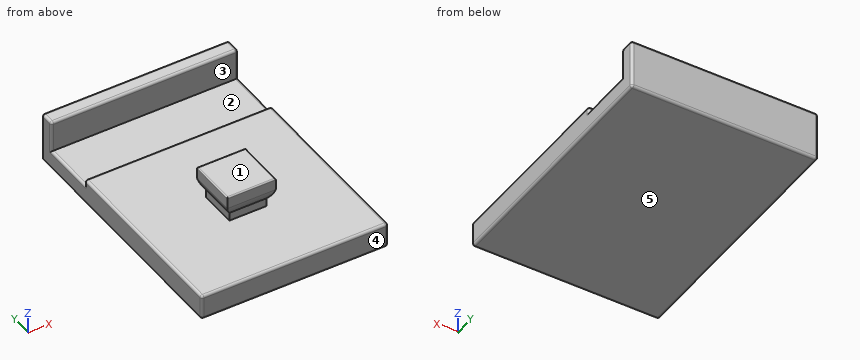
```python
from build123d import *

# Parameters (mm, degrees)
SKETCH_1_W                      = 15
SKETCH_1_H                      = 15
EXTRUDE_1_DEPTH                 = 2
SKETCH_2_W                      = 3
SKETCH_2_H                      = 3
EXTRUDE_2_DEPTH                 = 1
EXTRUDE_3_DEPTH                 = 2
EXTRUDE_3_DEPTH_BACK            = 2
CUT_EXTRUDE_1_REACH             = 12.897
CUT_EXTRUDE_1_DIRECTION_2_REACH = 12.897
FILLET_1_R                      = 0.1
SKETCH_5_W                      = 15
SKETCH_5_H                      = 1.5
EXTRUDE_4_DEPTH                 = 5.5
SKETCH_6_W                      = 15
SKETCH_6_H                      = 1.2
EXTRUDE_5_DEPTH                 = 2.5
FILLET_2_R                      = 0.2


with BuildPart() as part:
    # 草图1 → 凸台-拉伸1 (new body)
    with BuildSketch(Plane.XY):
        Rectangle(SKETCH_1_W, SKETCH_1_H)
    extrude(amount=-EXTRUDE_1_DEPTH)

    # 草图2 → 凸台-拉伸2 (add)
    with BuildSketch(Plane.XY):
        Rectangle(SKETCH_2_W, SKETCH_2_H)
    extrude(amount=EXTRUDE_2_DEPTH)

    # 草图3 → 凸台-拉伸3 (add, two sides: drawn at the far end of the back side and taken through both)
    with BuildSketch(Plane(origin=(0, 0, 0), x_dir=(1, 0, 0), z_dir=(0, 1, 0)).offset(-EXTRUDE_3_DEPTH_BACK)):
        with BuildLine():
            Line((-1.95, -2.5), (1.95, -2.5))
            Line((1.95, -2.5), (1.95, -1.555590279))
            ThreePointArc((1.95, -1.555590279), (1.780042303, -1.088161527), (1.5, -0.677124344))
            Line((1.5, -0.677124344), (-1.5, -0.677124344))
            ThreePointArc((-1.5, -0.677124344), (-1.780042303, -1.088161527), (-1.95, -1.555590279))
            Line((-1.95, -1.555590279), (-1.95, -2.5))
        make_face()
    extrude(amount=EXTRUDE_3_DEPTH + EXTRUDE_3_DEPTH_BACK)

    # 草图4 → 切除-拉伸1 (cut, up to next)
    with BuildSketch(Plane(origin=(0, 0, 0), x_dir=(0, 0, -1), z_dir=(1, 0, 0)), mode=Mode.PRIVATE) as cut_extrude_1_sk1:
        with BuildLine():
            Line((-2.5, 1.95), (-1.555590279, 1.95))
            ThreePointArc((-1.555590279, 1.95), (-1.088161527, 1.780042303), (-0.677124344, 1.5))
            Line((-0.677124344, 1.5), (-0.677124344, 2))
            Line((-0.677124344, 2), (-2.5, 2))
            Line((-2.5, 2), (-2.5, 1.95))
        make_face()
    cut_extrude_1_tool1 = extrude(cut_extrude_1_sk1.sketch, amount=-CUT_EXTRUDE_1_REACH, mode=Mode.PRIVATE) & part.part
    # 草图4 → 切除-拉伸1 (cut, up to next)
    with BuildSketch(Plane(origin=(0, 0, 0), x_dir=(0, 0, -1), z_dir=(1, 0, 0)), mode=Mode.PRIVATE) as cut_extrude_1_sk2:
        with BuildLine():
            Line((-2.5, -2), (-0.677124344, -2))
            Line((-0.677124344, -2), (-0.677124344, -1.5))
            ThreePointArc((-0.677124344, -1.5), (-1.088161527, -1.780042303), (-1.555590279, -1.95))
            Line((-1.555590279, -1.95), (-2.5, -1.95))
            Line((-2.5, -1.95), (-2.5, -2))
        make_face()
    cut_extrude_1_tool2 = extrude(cut_extrude_1_sk2.sketch, amount=-CUT_EXTRUDE_1_REACH, mode=Mode.PRIVATE) & part.part
    add(cut_extrude_1_tool1.solids().sort_by_distance((0, 1.873038, 1.175075))[0], mode=Mode.SUBTRACT)
    add(cut_extrude_1_tool2.solids().sort_by_distance((0, -1.873038, 1.175075))[0], mode=Mode.SUBTRACT)

    # 草图4 → 切除-拉伸1 direction 2 (cut, up to next)
    with BuildSketch(Plane(origin=(0, 0, 0), x_dir=(0, 0, -1), z_dir=(1, 0, 0)), mode=Mode.PRIVATE) as cut_extrude_1_direction_2_sk1:
        with BuildLine():
            Line((-2.5, 1.95), (-1.555590279, 1.95))
            ThreePointArc((-1.555590279, 1.95), (-1.088161527, 1.780042303), (-0.677124344, 1.5))
            Line((-0.677124344, 1.5), (-0.677124344, 2))
            Line((-0.677124344, 2), (-2.5, 2))
            Line((-2.5, 2), (-2.5, 1.95))
        make_face()
    cut_extrude_1_direction_2_tool1 = extrude(cut_extrude_1_direction_2_sk1.sketch, amount=CUT_EXTRUDE_1_DIRECTION_2_REACH, mode=Mode.PRIVATE) & part.part
    # 草图4 → 切除-拉伸1 direction 2 (cut, up to next)
    with BuildSketch(Plane(origin=(0, 0, 0), x_dir=(0, 0, -1), z_dir=(1, 0, 0)), mode=Mode.PRIVATE) as cut_extrude_1_direction_2_sk2:
        with BuildLine():
            Line((-2.5, -2), (-0.677124344, -2))
            Line((-0.677124344, -2), (-0.677124344, -1.5))
            ThreePointArc((-0.677124344, -1.5), (-1.088161527, -1.780042303), (-1.555590279, -1.95))
            Line((-1.555590279, -1.95), (-2.5, -1.95))
            Line((-2.5, -1.95), (-2.5, -2))
        make_face()
    cut_extrude_1_direction_2_tool2 = extrude(cut_extrude_1_direction_2_sk2.sketch, amount=CUT_EXTRUDE_1_DIRECTION_2_REACH, mode=Mode.PRIVATE) & part.part
    add(cut_extrude_1_direction_2_tool1.solids().sort_by_distance((0, 1.873038, 1.175075))[0], mode=Mode.SUBTRACT)
    add(cut_extrude_1_direction_2_tool2.solids().sort_by_distance((0, -1.873038, 1.175075))[0], mode=Mode.SUBTRACT)

    # 圆角1
    fillet_1_edges = [part.edges().sort_by_distance(p)[0] for p in [
        (-1.95, 0, 2.5),
        (1.95, 0, 2.5),
        (0, -1.95, 2.5),
        (0, 1.95, 2.5),
    ]]
    fillet(fillet_1_edges, radius=FILLET_1_R)

    # 草图5 → 凸台-拉伸4 (add)
    with BuildSketch(Plane(origin=(0, 7.5, 0), x_dir=(1, 0, 0), z_dir=(0, 1, 0))):
        with Locations((0, 1.25)):
            Rectangle(SKETCH_5_W, SKETCH_5_H)
    extrude(amount=EXTRUDE_4_DEPTH)

    # 草图6 → 凸台-拉伸5 (add)
    with BuildSketch(Plane.XY.offset(-0.5)):
        with Locations((0, 12.4)):
            Rectangle(SKETCH_6_W, SKETCH_6_H)
    extrude(amount=EXTRUDE_5_DEPTH)

    # 圆角2
    fillet_2_edges = [part.edges().sort_by_distance(p)[0] for p in [
        (0, -7.5, -2),
        (0, -7.5, 0),
        (-7.5, -7.5, -1),
        (-7.5, 2.75, -2),
        (-7.5, 12.4, 2),
        (-7.5, 11.8, 0.75),
        (-7.5, 9.65, -0.5),
        (-7.5, 7.5, -0.25),
        (-7.5, 0, 0),
        (7.5, 7.5, -0.25),
        (7.5, 9.65, -0.5),
        (7.5, 11.8, 0.75),
        (7.5, 12.4, 2),
        (7.5, 2.75, -2),
        (7.5, -7.5, -1),
        (7.5, 0, 0),
        (0, 13, -2),
        (7.5, 13, 0),
        (0, 13, 2),
        (-7.5, 13, 0),
        (0, 7.5, 0),
        (0, 11.8, 2),
    ]]
    fillet(fillet_2_edges, radius=FILLET_2_R)


solid = part.part
```
The model under review builds one solid part; all positions refer to its coordinate system, in mm. Face numbers are marked on the shaded views. A direction names the side the tool comes from. Coordinates: 2 decimals unless noted, no trailing zeros. Write each loop counter-clockwise with the first axis right and the second up, starting at its lowest first coordinate (ties: lowest second). Pieces come first, ordered by that corner, then holes.
1) The part is to be moulded in two halves that separate along Y. For the marked faces 3, 4 and 5, say which applies: pulls with the +Y half, pulls with the -Y half, needs draft (parallel to the pull), parting line crosses it, or undercut.
2) We need section B-B on y = -0.5. State the section outline as (x, z) points, then the cut area to 3 significant figures.
3) Machinability: for the marked faces 1 and 2, which of the approach directions +Z, -Z, +X, -X, +Y, -Y give a long, thin tool a straight path to every point of the face, cutting with its end or side? Answer none if there is none.
4) To check wall thickness, follow probe 1 along Y at (x, z) = (-1.75, 1.7); probe 2 along Y at (x, z) = (0.75, 0.3); probe 3 along Z at (x, y) = (-7, 3.5). State the ranges of each line that lie inside material, in increasing order.
5) Clearance check with flat-ended pins moving along their axes: pin 1 Ø1.3 at (x, y) = (2, 10) entering from +Z; pin 2 Ø1 at (x, y) = (5.5, 2.5) entering from +Z; pin 3 Ø1 at (y, z) = (7.5, 1.5) entering from +X; pin 4 Ø0.9 at (x, z) = (0, 2) entering from -Y. State where each tip first meets the part, or that it passes through.
6) We need section A-A on z = 0.45. State the section outline as (x, y) points, then the cut area to 3 significant figures.
7) We need section D-D on y = 3.25. State the section outline as (x, z) points.
8) We need section C-C on x = 6.5. State the section outline as (y, z) points.
Answer list:
1. face 3: undercut
1. face 4: pulls with the -Y half
1. face 5: needs draft
2. outline: (-7.5, -1.8) arc R0.2 ccw to (-7.3, -2) - (7.3, -2) arc R0.2 ccw to (7.5, -1.8) - (7.5, -0.2) arc R0.2 ccw to (7.3, 0) - (1.5, 0) - (1.5, 0.68) arc R2 ccw to (1.95, 1.56) - (1.95, 2.4) arc R0.1 ccw to (1.85, 2.5) - (-1.85, 2.5) arc R0.1 ccw to (-1.95, 2.4) - (-1.95, 1.56) arc R2 ccw to (-1.5, 0.68) - (-1.5, 0) - (-7.3, 0) arc R0.2 ccw to (-7.5, -0.2) - close
2. area: 38.8 mm2
3. face 1: +Z, +X, -X, +Y, -Y
3. face 2: +Z, +X, -X
4. probe 1: y = -1.95 to 1.95, 11.8 to 13
4. probe 2: y = -1.5 to 1.5, 11.8 to 13
4. probe 3: z = -2 to 0
5. pin 1: stops at z = -0.5
5. pin 2: stops at z = 0
5. pin 3: passes through
5. pin 4: stops at y = -1.95
6. outline: (-7.5, 12) arc R0.2 ccw to (-7.3, 11.8) - (7.3, 11.8) arc R0.2 ccw to (7.5, 12) - (7.5, 12.8) arc R0.2 ccw to (7.3, 13) - (-7.3, 13) arc R0.2 ccw to (-7.5, 12.8) - close; (-1.5, -1.5) - (1.5, -1.5) - (1.5, 1.5) - (-1.5, 1.5) - close
6. area: 27.0 mm2
7. outline: (-7.5, -1.8) arc R0.2 ccw to (-7.3, -2) - (7.3, -2) arc R0.2 ccw to (7.5, -1.8) - (7.5, -0.2) arc R0.2 ccw to (7.3, 0) - (-7.3, 0) arc R0.2 ccw to (-7.5, -0.2) - close
8. outline: (-7.5, -1.8) arc R0.2 ccw to (-7.3, -2) - (12.8, -2) arc R0.2 ccw to (13, -1.8) - (13, 1.8) arc R0.2 ccw to (12.8, 2) - (12, 2) arc R0.2 ccw to (11.8, 1.8) - (11.8, -0.5) - (7.5, -0.5) - (7.5, -0.2) arc R0.2 ccw to (7.3, 0) - (-7.3, 0) arc R0.2 ccw to (-7.5, -0.2) - close
